For this review, take the finished solid that the model builds, in its own axes (mm). A direction names the side the tool comes from. Give positions to 0.01 mm unless a question says otherwise; leave off trailing zeros. Order: outer loops, then holes, each group sorted by start corner. A loop starts at its lowest first (then second) coordinate and runs counter-clockwise, first axis right, second up. Notation, with made-up numbers: (74, 65) -> (93, 65) arc R27 cw to (93, 88) -> close; hole circle Ø10 at (-37, 77.5). An arc over 180 degrees is marked (long way). Return JSON: item names as keys, results as strings. Group by question number.
1) For faces 4 (the face through (18.722, 0.066, 7.965)), 5 (the face through (25, 29, 4)), 6 (the face through (-19.05, -26, 28)), 7 (the face through (-28, -16, 10)), 8 (the face through (-18.9, 1.2, 10.5)), list the 3-axis set-ups (+Z, -Z, +X, -X, +Y, -Y) from which the entire face can be reached by the end or side of a thin tool; tool diameter is ignored.
2) Add section B-B (z = 47.5). Give the boundary of the cut face in (x, y).
3) To check wall thickness, follow line 1 along Y through (x, z) = (-21, 30.5); line 2 along Z through (x, y) = (2.5, -25.5); line 3 along X through (y, z) = (10.5, 46.5). State the ranges of each line that lie inside material, in increasing order.
4) Insertion check: P1, Ø2, axis at x = -10, y = 15.5, coming from the +Z side; P2, Ø4, axis at x = 27, y = -33.5, coming from the +Z side; P3, Ø1, axis at x = -28, z = 7, coming from the +Y side. Each pin has a flat end and moves straight along its axis. Give the tip position at first contact, or say it passes through.
5) Add section C-C (x = -8). Give the boundary of the cut face in (y, z).
6) Add section A-A (y = 32.5). Give the boundary of the cut face in (x, z).
7) The part is to be moulded in two halves that separate along Y. For faces 1 (the face through (0, 0, 3.5)), 2 (the face through (19.05, -26, 27)), 3 (the face through (-0.207, -14.452, 4.755)), say which applies: released by +Y, released by -Y, zero draft, split by the parting line, or undercut.
8) Add section D-D (y = 9.5). Give the boundary of the cut face in (x, z), then the cut area to 3 significant figures.
from build123d import *

# Parameters (mm, degrees)
F0_W            = 60
F0_H            = 55
F1_DEPTH        = 55
F2_T            = -3.5
F4_DEPTH        = 5
F6_D            = 3
F6_DEPTH        = 12
F6_TIP          = 0.9012909285
F8_D            = 3
F8_DEPTH        = 12
F8_TIP          = 0.9012909285
F7_W            = 41
F7_H            = 35
F9_DEPTH        = 25
F10_R           = 5
F11_DEPTH       = 7
F13_D           = 3
F13_DEPTH       = 5
F13_TIP         = 0.9012909285
F14_W           = 7
F14_H           = 3
F15_DEPTH       = 5
F16_W           = 7
F16_H           = 5
F17_DEPTH       = 5
F18_W           = 24
F18_H           = 6
F19_DEPTH       = 4
F21_D           = 3
F21_DEPTH       = 5
F21_TIP         = 0.9012909285
F23_D           = 3
F23_DEPTH       = 5
F23_TIP         = 0.9012909285
F24_W           = 5
F24_H           = 10
F25_DEPTH       = 10
F27_D           = 3.3
F27_DEPTH       = 5
F27_CSINK_D     = 6.72
F27_CSINK_ANGLE = 90
F27_TIP         = 0.9914200214
F28_W           = 5
F28_H           = 10
F29_DEPTH       = 10
F31_D           = 3.3
F31_DEPTH       = 5
F31_CSINK_D     = 6.72
F31_CSINK_ANGLE = 90
F31_TIP         = 0.9914200214


with BuildPart() as f1:
    # F0 (on Top) → F1 (new body)
    with BuildSketch(Plane.XY):
        Rectangle(F0_W, F0_H)
    extrude(amount=F1_DEPTH)

    # F2
    f2_openings = [f1.faces().sort_by_distance(p)[0] for p in [
        (0, 0, 55),
    ]]
    offset(amount=F2_T, openings=f2_openings)

    # F3 (on face) → F4 (cut)
    with BuildSketch(Plane.XZ.offset(27.5)):
        Polygon((19.05, 39.8), (-19.05, 39.8), (-19.05, 15.2), (0, 15.2), (19.05, 15.2), align=None)
    extrude(amount=-F4_DEPTH, mode=Mode.SUBTRACT)

    # F6
    with Locations(Plane.XZ.offset(27.5)):
        with Locations((-21.8598913223, 37.825), (-21.8598913223, 17.175), (21.5401086777, 17.175), (21.5401086777, 37.825)):
            Hole(F6_D / 2, depth=F6_DEPTH)
            with Locations((0, 0, -(F6_DEPTH + F6_TIP / 2))):  # 118° drill point
                Cone(0, F6_D / 2, F6_TIP, mode=Mode.SUBTRACT)

    # F8
    with Locations(Plane(origin=(-30, 0, 0), x_dir=(0, -1, 0), z_dir=(-1, 0, 0))):
        with Locations((-20, 47.5), (-20, 7.5), (20, 7.5), (20, 47.5)):
            Hole(F8_D / 2, depth=F8_DEPTH)
            with Locations((0, 0, -(F8_DEPTH + F8_TIP / 2))):  # 118° drill point
                Cone(0, F8_D / 2, F8_TIP, mode=Mode.SUBTRACT)

    # F7 (on face) → F9 (cut)
    with BuildSketch(Plane(origin=(-30, 0, 0), x_dir=(0, -1, 0), z_dir=(-1, 0, 0))):
        with Locations((0, 27.5)):
            Rectangle(F7_W, F7_H)
    extrude(amount=-F9_DEPTH, mode=Mode.SUBTRACT)

    # F10 (on face) → F11 (join)
    with BuildSketch(Plane.XY.offset(3.5)):
        with Locations((-17.7631583065, 0)):
            Circle(F10_R)
        with Locations((0, 15.3929423541)):
            Circle(F10_R)
        with Locations((16.9736854732, 0)):
            Circle(F10_R)
        with Locations((0, -14.607058838)):
            Circle(F10_R)
    extrude(amount=F11_DEPTH)

    # F13
    with Locations(Plane.XY.offset(10.5)):
        with Locations((0, 15.4706398025), (-17.7631583065, 0), (0, -14.2931165174), (17.22384803, 0)):
            Hole(F13_D / 2, depth=F13_DEPTH)
            with Locations((0, 0, -(F13_DEPTH + F13_TIP / 2))):  # 118° drill point
                Cone(0, F13_D / 2, F13_TIP, mode=Mode.SUBTRACT)

    # F14 (on face) → F15 (cut)
    with BuildSketch(Plane.YZ.offset(30)):
        with Locations((0, 28.8139954209)):
            Rectangle(F14_W, F14_H)
    extrude(amount=-F15_DEPTH, mode=Mode.SUBTRACT)

    # F16 (on face) → F17 (cut)
    with BuildSketch(Plane(origin=(0, 27.5, 0), x_dir=(-1, 0, 0), z_dir=(0, 1, 0))):
        with Locations((0, 29.2087327689)):
            Rectangle(F16_W, F16_H)
    extrude(amount=-F17_DEPTH, mode=Mode.SUBTRACT)

    # F18 (on face) → F19 (cut)
    with BuildSketch(Plane(origin=(-30, 0, 0), x_dir=(0, -1, 0), z_dir=(-1, 0, 0))):
        with Locations((0, 7)):
            Rectangle(F18_W, F18_H)
    extrude(amount=-F19_DEPTH, mode=Mode.SUBTRACT)

    # F21
    with Locations(Plane.YZ.offset(30)):
        with Locations((0, 43.075658381), (0, 14.3585540354)):
            Hole(F21_D / 2, depth=F21_DEPTH)
            with Locations((0, 0, -(F21_DEPTH + F21_TIP / 2))):  # 118° drill point
                Cone(0, F21_D / 2, F21_TIP, mode=Mode.SUBTRACT)

    # F23
    with Locations(Plane(origin=(0, 27.5, 0), x_dir=(-1, 0, 0), z_dir=(0, 1, 0))):
        with Locations((0, 37.1811050391), (0, 13.7660141307)):
            Hole(F23_D / 2, depth=F23_DEPTH)
            with Locations((0, 0, -(F23_DEPTH + F23_TIP / 2))):  # 118° drill point
                Cone(0, F23_D / 2, F23_TIP, mode=Mode.SUBTRACT)

    # F24 (on face) → F25 (join)
    with BuildSketch(Plane.XZ.offset(27.5)):
        with Locations((27.5, 5)):
            Rectangle(F24_W, F24_H)
    extrude(amount=F25_DEPTH)

    # F27
    with Locations(Plane(origin=(25, 0, 0), x_dir=(0, -1, 0), z_dir=(-1, 0, 0))):
        with Locations((32.5, 5)):
            CounterSinkHole(F27_D / 2, F27_CSINK_D / 2, depth=F27_DEPTH, counter_sink_angle=F27_CSINK_ANGLE)
            with Locations((0, 0, -(F27_DEPTH + F27_TIP / 2))):  # 118° drill point
                Cone(0, F27_D / 2, F27_TIP, mode=Mode.SUBTRACT)

    # F28 (on face) → F29 (join)
    with BuildSketch(Plane(origin=(0, 27.5, 0), x_dir=(-1, 0, 0), z_dir=(0, 1, 0))):
        with Locations((-27.5, 5)):
            Rectangle(F28_W, F28_H)
    extrude(amount=F29_DEPTH)

    # F31
    with Locations(Plane(origin=(25, 0, 0), x_dir=(0, -1, 0), z_dir=(-1, 0, 0))):
        with Locations((-32.5, 5)):
            CounterSinkHole(F31_D / 2, F31_CSINK_D / 2, depth=F31_DEPTH, counter_sink_angle=F31_CSINK_ANGLE)
            with Locations((0, 0, -(F31_DEPTH + F31_TIP / 2))):  # 118° drill point
                Cone(0, F31_D / 2, F31_TIP, mode=Mode.SUBTRACT)


solid = f1.part
Evaluation:
{
 "1": {"face 4": "+Z", "face 5": "+Z, -Z, -X, +Y", "face 6": "-Y", "face 7": "-X", "face 8": "+Z, -X"},
 "2": {"outline": "(-30, -27.5) -> (30, -27.5) -> (30, 27.5) -> (-30, 27.5) -> (-30, 21.5) -> (-26.5, 21.5) -> (-26.5, 24) -> (26.5, 24) -> (26.5, -24) -> (-26.5, -24) -> (-26.5, -21.5) -> (-30, -21.5) -> close; (-30, -18.5) -> (-26.5, -18.5) -> (-26.5, 18.5) -> (-30, 18.5) -> close"},
 "3": {"line 1": "-27.5 to -24, 24 to 27.5", "line 2": "0 to 15.2, 39.8 to 55", "line 3": "-30 to -26.5, 26.5 to 30"},
 "4": {"P1": "z = 3.5", "P2": "z = 10", "P3": "y = 27.5"},
 "5": {"outline": "(-27.5, 0) -> (27.5, 0) -> (27.5, 55) -> (24, 55) -> (24, 3.5) -> (-24, 3.5) -> (-24, 15.2) -> (-27.5, 15.2) -> close; (-27.5, 39.8) -> (-24, 39.8) -> (-24, 55) -> (-27.5, 55) -> close"},
 "6": {"outline": "(25, 0) -> (30, 0) -> (30, 3.35) -> (26.71, 3.35) -> (25, 1.64) -> close; (25, 8.36) -> (26.71, 6.65) -> (30, 6.65) -> (30, 10) -> (25, 10) -> close"},
 "7": {"face 1": "undercut", "face 2": "zero draft", "face 3": "undercut"},
 "8": {"outline": "(-30, 0) -> (30, 0) -> (30, 55) -> (26.5, 55) -> (26.5, 3.5) -> (-26.5, 3.5) -> (-26.5, 4) -> (-30, 4) -> close; (-30, 45) -> (-26.5, 45) -> (-26.5, 55) -> (-30, 55) -> close", "area": "427 mm^2"}
}
